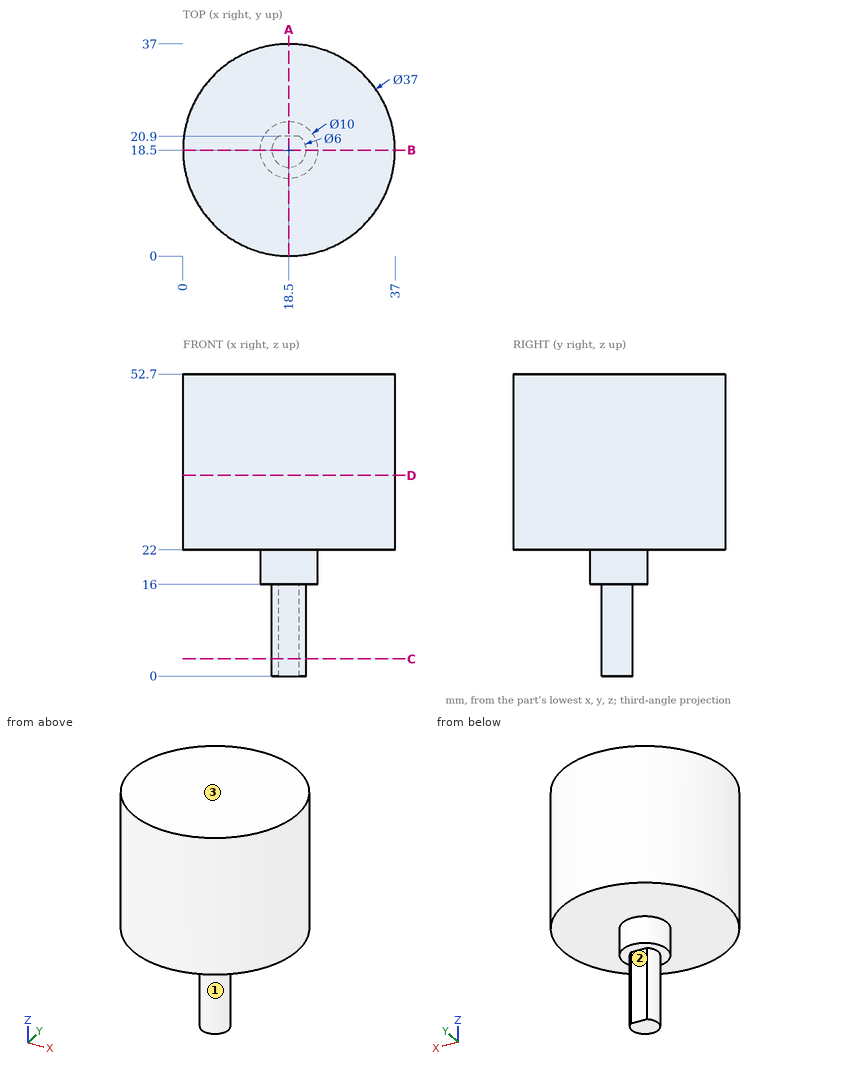
Design review of the part shown in the three views and the two pictorial views. Dimensions are in mm from the part's minimum x, y and z. A direction names the side the tool comes from. Give positions to 0.01 mm unless a question says otherwise; leave off trailing zeros. Order: outer loops, then holes, each group sorted by start corner. A loop starts at its lowest first (then second) coordinate and runs counter-clockwise, first axis right, second up. Notation, with made-up numbers: (83, -7.5) -> (111, -7.5) arc R21 ccw to (111, 10.5) -> close; hole circle Ø9 at (-0.5, 28.25). An arc over 180 degrees is marked (long way). Write each question's results on one line, items separated by ' | '. Start each with the question number.
Q1. For pin 1 (6 mm diameter, centred on y = 7, z = 23, fed in from +X); pin 2 (3 mm diameter, centred on y = 27, z = 44, fed in from +X); pin 3 (6 mm diameter, centred on y = 25, z = 37.5, fed in from -X), all flat-tipped, find the tip position at first contact; note any pin that passes through.
Q2. Machinability: for the marked faces 1, 2 and 3, which of the approach directions +Z, -Z, +X, -X, +Y, -Y give a long, thin tool a straight path to every point of the face, cutting with its end or side? Answer none if there is none.
Q3. Add section A-A on x = 18.5. Give the boundary of the cut face in (y, z).
Q4. Wall thickness on L1, parallel to Z at x = 16.5, y = 7; L2, parallel to X at y = 13.5, z = 27; L3, parallel to Y at x = 3.5, z = 38: over which ranges is each line inside the solid? List them lowest first. Write a range as from..to.
Q5. Add section D-D on z = 35. Give the boundary of the cut face in (x, y), and give its area (3 significant figures).
Q6. Add section B-B on y = 18.5. Give the boundary of the cut face in (x, z), and give its area (3 significant figures).
Q7. Add section C-C on z = 3. Give the boundary of the cut face in (x, y), and give its area (3 significant figures).
Found:
1) pin 1: stops at x = 34.93 | pin 2: stops at x = 35.62 | pin 3: stops at x = 0.33
2) face 1: -Z | face 2: -Z, +X, -X, +Y | face 3: +Z, +X, -X, +Y, -Y
3) outline: (0, 22) -> (13.5, 22) -> (13.5, 16) -> (15.5, 16) -> (15.5, 0) -> (20.9, 0) -> (20.9, 16) -> (23.5, 16) -> (23.5, 22) -> (37, 22) -> (37, 52.7) -> (0, 52.7) -> close
4) L1: z = 22..52.7 | L2: x = 0.69..36.31 | L3: y = 7.67..29.33
5) outline: circle Ø37 at (18.5, 18.5) | area: 1,080 mm2
6) outline: (0, 22) -> (13.5, 22) -> (13.5, 16) -> (15.5, 16) -> (15.5, 0) -> (21.5, 0) -> (21.5, 16) -> (23.5, 16) -> (23.5, 22) -> (37, 22) -> (37, 52.7) -> (0, 52.7) -> close | area: 1,290 mm2
7) outline: (16.7, 20.9) arc R3 ccw (long way) to (20.3, 20.9) -> close | area: 26.8 mm2
